Autodesk Inventor part; units mm, degrees
ref_plane "YZ Plane" through (0, 0, 0) normal (1, 0, 0) x (0, 1, 0)
ref_plane "XZ Plane" through (0, 0, 0) normal (0, 1, 0) x (-1, 0, 0)
ref_plane "XY Plane" through (0, 0, 0) normal (0, 0, 1) x (1, 0, 0)
ref_plane "作業平面1" through (15.3757, 45.25, -5) normal (0, 0, -1) x (-1, 0, 0)
sketch "Base_plate" plane through (15.3757, 45.25, -5) normal (0, 0, -1) x (-1, 0, 0)
  circle A0 centre (-112.6243, -12.25) radius 3.25
  circle A1 centre (-112.6243, -78.25) radius 3.25
  circle A2 centre (143.3757, -78.25) radius 3.25
  circle A3 centre (143.3757, -12.25) radius 3.25
  line L0 (151.578, -11.3644) -> (151.578, -77.3644)
  arc A4 (151.578, -11.3644) -> (147.5007, -5.1053) centre (143.3757, -12.25) ccw
  line L1 (147.5007, -5.1053) -> (140.9785, -1.3397)
  arc A5 (140.9785, -1.3397) -> (135.9785, 0) centre (135.9785, -10) ccw
  line L2 (135.9785, 0) -> (0, 0)
  line L3 (-20.2421, 7.2915) -> (-3.697, 0.7085)
  line L4 (-23.9391, 8) -> (-103.3743, 8)
  line L5 (0, 0) -> (135.9785, 0)
  arc A6 (140.9785, -1.3397) -> (135.9785, 0) centre (135.9785, -10) ccw
  line L6 (140.9785, -1.3397) -> (147.5007, -5.1053)
  arc A7 (151.578, -11.3644) -> (147.5007, -5.1053) centre (143.3757, -12.25) ccw
  line L7 (151.578, -11.3644) -> (151.578, -77.3644)
  arc A8 (147.5007, -85.3947) -> (151.578, -77.3644) centre (143.3757, -78.25) ccw
  arc A9 (-103.3743, 8) -> (-111.5876, 3.7046) centre (-103.3743, -2) ccw
  line L8 (-103.3743, 8) -> (-23.9391, 8)
  arc A10 (-20.2421, 7.2915) -> (-23.9391, 8) centre (-23.9391, -2) ccw
  line L9 (-20.2421, 7.2915) -> (-3.697, 0.7085)
  arc A11 (-3.697, 0.7085) -> (0, 0) centre (0, 10) ccw
  circle A12 centre (-112.6243, -12.25) radius 3.25
  circle A13 centre (143.3757, -12.25) radius 3.25
  circle A14 centre (143.3757, -78.25) radius 3.25
  circle A15 centre (-112.6243, -78.25) radius 3.25
  line L10 (135.9785, 0) -> (0, 0)
  arc A16 (140.9785, -1.3397) -> (135.9785, 0) centre (135.9785, -10) ccw
  line L11 (147.5007, -5.1053) -> (140.9785, -1.3397)
  arc A17 (151.578, -11.3644) -> (147.5007, -5.1053) centre (143.3757, -12.25) ccw
  line L12 (151.6257, -11.3644) -> (151.6257, -77.3644)
  arc A18 (147.5007, -85.3947) -> (151.578, -77.3644) centre (143.3757, -78.25) ccw
  line L13 (147.5007, -85.3947) -> (140.9785, -89.1603)
  arc A19 (135.9785, -90.5) -> (140.9785, -89.1603) centre (135.9785, -80.5) ccw
  line L14 (135.9785, -90.5) -> (0, -90.5)
  arc A20 (0, -90.5) -> (-3.697, -91.2085) centre (0, -100.5) ccw
  line L15 (-20.2421, -97.7915) -> (-3.697, -91.2085)
  arc A21 (-23.9391, -98.5) -> (-20.2421, -97.7915) centre (-23.9391, -88.5) ccw
  line L16 (-23.9391, -98.5) -> (-103.3743, -98.5)
  arc A22 (-111.5876, -94.2046) -> (-103.3743, -98.5) centre (-103.3743, -88.5) ccw
  line L17 (-111.5876, -94.2046) -> (-119.4003, -82.9563)
  arc A23 (-120.8743, -78.25) -> (-119.4003, -82.9563) centre (-112.6243, -78.25) ccw
  line L18 (-120.8743, -12.25) -> (-120.8743, -78.25)
  arc A24 (-119.4003, -7.5437) -> (-120.8743, -12.25) centre (-112.6243, -12.25) ccw
  line L19 (-111.5876, 3.7046) -> (-119.4003, -7.5437)
  line L20 (-23.9391, 8) -> (-103.3743, 8)
  arc A25 (-20.2421, 7.2915) -> (-23.9391, 8) centre (-23.9391, -2) ccw
  line L21 (-20.2421, 7.2915) -> (-3.697, 0.7085)
  arc A26 (-3.697, 0.7085) -> (0, 0) centre (0, 10) ccw
  line L22 (101.578, 7.8213) -> (101.578, -100.5) construction
  line L23 (151.6257, -44.3644) -> (-114.4175, -44.3644) construction
  circle A27 centre (56.078, -44.3644) radius 17.5 construction
  line L24 (129.578, -5.1053) -> (129.578, -82.9563) construction
  circle A28 centre (129.578, -16.3644) radius 1.75
  circle A29 centre (129.578, -72.3644) radius 1.75
  line L25 (59.578, -19.3302) -> (59.578, -75) construction
  circle A30 centre (59.578, -24.3644) radius 1.75
  circle A31 centre (59.578, -64.3644) radius 1.75
  circle A32 centre (101.578, -44.3644) radius 14.75 construction
  line L26 (101.578, -44.3644) -> (118.6401, -27.3023) construction
  line L27 (101.578, -44.3644) -> (125.7075, -44.3644) construction
  line L28 (106.5779, -39.3645) -> (117.1845, -28.7579) construction
  line L29 (107.7093, -40.4959) -> (118.3159, -29.8893)
  line L30 (116.0532, -27.6265) -> (105.4466, -38.2331)
  arc A33 (105.4466, -38.2331) -> (107.7093, -40.4959) centre (106.5779, -39.3645) ccw
  arc A34 (118.3159, -29.8893) -> (116.0532, -27.6265) centre (117.1845, -28.7579) ccw
  line L31 (84.8401, -29.8893) -> (95.4467, -40.4959)
  arc A35 (87.1028, -27.6265) -> (84.8401, -29.8893) centre (85.9714, -28.7579) ccw
  line L32 (97.7094, -38.2331) -> (87.1028, -27.6265)
  arc A36 (95.4467, -40.4959) -> (97.7094, -38.2331) centre (96.578, -39.3645) ccw
  line L33 (87.1028, -61.1024) -> (97.7094, -50.4958)
  arc A37 (84.8401, -58.8396) -> (87.1028, -61.1024) centre (85.9714, -59.971) ccw
  line L34 (95.4467, -48.233) -> (84.8401, -58.8396)
  arc A38 (97.7094, -50.4958) -> (95.4467, -48.233) centre (96.578, -49.3644) ccw
  line L35 (118.3159, -58.8396) -> (107.7093, -48.233)
  arc A39 (116.0532, -61.1024) -> (118.3159, -58.8396) centre (117.1845, -59.971) ccw
  line L36 (105.4466, -50.4958) -> (116.0532, -61.1024)
  arc A40 (107.7093, -48.233) -> (105.4466, -50.4958) centre (106.5779, -49.3644) ccw
  line L37 (65.0919, -29.3644) -> (74.078, -29.3644)
  line L38 (84.078, -39.3644) -> (84.078, -49.3644)
  line L39 (74.078, -59.3644) -> (65.0919, -59.3644)
  line L40 (65.0919, -59.3644) -> (65.0919, -29.3644) construction
  arc A41 (84.078, -39.3644) -> (74.078, -29.3644) centre (74.078, -39.3644) ccw
  arc A42 (74.078, -59.3644) -> (84.078, -49.3644) centre (74.078, -49.3644) ccw
  arc A43 (65.0919, -29.3644) -> (65.0919, -59.3644) centre (56.078, -44.3644) ccw
  line L41 (-60.8743, -12.5765) -> (-60.8743, -79.1684) construction
  line L42 (-98.3743, -6.8644) -> (-23.3743, -6.8644) construction
  line L43 (-23.3743, -6.8644) -> (-23.3743, -81.8644) construction
  line L44 (-23.3743, -81.8644) -> (-98.3743, -81.8644) construction
  line L45 (-98.3743, -81.8644) -> (-98.3743, -6.8644) construction
  line L46 (-98.3743, -6.8644) -> (-23.3743, -81.8644) construction
  line L47 (-23.3743, -6.8644) -> (-98.3743, -81.8644) construction
  circle A44 centre (-98.3743, -6.8644) radius 2.1
  circle A45 centre (-23.3743, -6.8644) radius 2.1
  circle A46 centre (-98.3743, -81.8644) radius 2.1
  circle A47 centre (-23.3743, -81.8644) radius 2.1
  point P0 (144.2396, -3.2225)
  point P1 (144.2396, -87.2775)
  point P2 (111.8812, -34.0612)
  point P3 (91.2747, -34.0612)
  point P4 (91.2747, -54.6677)
  point P5 (111.8812, -54.6677)
  point P6 (-60.8743, -44.3644)
  point P7 (-60.8743, -44.3644)
  dimension "d20" = 50
  dimension "d21" = 45.5
  dimension "d22" = 35
  dimension "d23" = 28
  dimension "d24" = 3.5
  dimension "d25" = 3.5
  dimension "d26" = 28
  dimension "d27" = 28
  dimension "d28" = 42
  dimension "d29" = 3.5
  dimension "d30" = 3.5
  dimension "d31" = 20
  dimension "d32" = 20
  dimension "d40" = 29.5
  dimension "d43" = 45
  dimension "d44" = 3.2
  dimension "d45" = 7.071
  dimension "d46" = 15
  dimension "d49" = 360
  dimension "d51" = 15
  dimension "d52" = 15
  dimension "d53" = 28
  dimension "d54" = 10
  dimension "d65" = 60
  dimension "d66" = 75
  dimension "d67" = 75
  dimension "d68" = 4.2
  dimension "d69" = 4.2
  dimension "d70" = 4.2
  dimension "d71" = 4.2
sketch "RPLidarA1M8" plane through (15.3757, 45.25, -5) normal (0, 0, -1) x (-1, 0, 0)
  line L0 (59.578, -45.9195) -> (59.578, -117.33) construction
  circle A0 centre (59.578, -24.3644) radius 1.5
  circle A1 centre (59.578, -64.3644) radius 1.5
  line L1 (4.0197, -44.3644) -> (199.1363, -44.3644) construction
  circle A2 centre (129.578, -16.3644) radius 1.5
  line L2 (101.578, -2.732) -> (101.578, -85.9969) construction
  circle A3 centre (101.578, -44.3644) radius 35.14
  line L3 (59.578, -6.852) -> (59.578, -81.8768) construction
  circle A4 centre (129.578, -72.3644) radius 1.5
  line L4 (129.578, -10.2254) -> (129.578, -77.75) construction
  circle A5 centre (56.078, -44.3644) radius 10
  circle A6 centre (56.078, -44.3644) radius 16
  line L5 (151.6257, -44.3644) -> (-114.4175, -44.3644) construction
  line L6 (101.578, 7.8213) -> (101.578, -100.5) construction
  point P0 (15.3757, -88.1377)
  point P1 (59.578, -44.3644)
  point P2 (129.578, -43.9877)
  dimension "d1" = 3
  dimension "d2" = 3
  dimension "d5" = 20
  dimension "d6" = 3
  dimension "d10" = 70.28
  dimension "d11" = 42
  dimension "d12" = 40
  dimension "d13" = 3
  dimension "d14" = 28
  dimension "d15" = 28
  dimension "d16" = 28
  dimension "d17" = 20
  dimension "d18" = 45.5
  dimension "d19" = 32
sketch "RPLidarA2M6" plane through (15.3757, 45.25, -5) normal (0, 0, -1) x (-1, 0, 0)
  line L0 (101.578, 7.8213) -> (101.578, -100.5) construction
  line L1 (151.6257, -44.3644) -> (-114.4175, -44.3644) construction
  circle A0 centre (101.578, -44.3644) radius 14.75 construction
  circle A1 centre (112.0078, -33.9346) radius 1.5
  line L2 (112.0078, -33.9346) -> (101.578, -44.3644) construction
  circle A2 centre (91.1482, -33.9346) radius 1.5
  circle A3 centre (91.1482, -54.7943) radius 1.5
  circle A4 centre (112.0078, -54.7943) radius 1.5
  dimension "d33" = 29.5
  dimension "d34" = 3
  dimension "d35" = 45
  dimension "d38" = 360
extrude "押し出し1" add sketch "Base_plate" along normal blind 5
Read the model definition and answer for the solid it produces. Units are mm, in the model's axes. A direction names the side the tool comes from. Coordinates: 2 decimals unless noted, no trailing zeros. Loops run counter-clockwise (first coordinate to the right, second up) from the corner with the lowest first, then second, coordinate; pieces in that order, holes last. Notation, with made-up numbers: (-17.5, -37) -> (-1.5, -37) arc R17 cw to (-1.5, -21) -> close; hole circle Ø9 at (81.25, 51). An arc over 180 degrees is marked (long way). Write item = value, one per line. Start each with the question number.
1) The part is cut by section B-B, the plane y = 11.5. Determine the outline of the cut face in (x, z), plus the area to 3 significant figures.
2) The mould has two halves that part along Y. Classify faces 1 (the face through (-134.88, 37.55, -7.46)), 2 (the face through (-131.002, -31.755, -7.465)), 3 (the face through (27.461, -49.296, -7.465)): pulls with the +Y half, pulls with the -Y half, needs draft (parallel to the pull), parting line crosses it, or undercut.
3) The part is cut by section A-A, the plane x = -128. Determine the outline of the cut face in (y, z).
4) Given P1, Ø4, axis at x = -128, y = 33, coming from the -Z side; P2, Ø5, axis at x = 38.75, y = 38.39, coming from the +Z side; P3, Ø2.5, axis at x = -28, z = -8.5, coming from the -Y side; P4, Ø2, axis at x = 12.5, z = -9, coming from the +Y side, each flat-ended and moving along its own axis, determine where each tip first touches the part or whether it passes through.
5) The part is cut by section C-C, the plane x = -28.5. Determine the outline of the cut face in (y, z), plus the area to 3 significant figures.
6) For faces 4 (the face through (-68.702, 1, -7)), 5 (the face through (-123.156, 44.919, -7.465)), determine the directions among +Z, -Z, +X, -X, +Y, -Y from which every point of the face is accessible in a straight line to the end or side of a thin tool.
7) Find the intervals of material crossed by L1, parallel to Y at x = 113.75, z = -6.4; L2, parallel to Y at x = -101, z = -7.1; L3, parallel to X at y = -6, z = -9.25, in increasing order. Write a range as from..to.
8) The part is cut by section D-D, the plane z = -6.75. State how many separate pieces and enclosed holes the cut face has, plus the area to 3 significant figures.
Result:
q1.outline = (-136.2, -10) -> (-99.08, -10) -> (-99.08, -5) -> (-136.2, -5) -> close; (-94.55, -10) -> (-77.85, -10) -> (-77.85, -5) -> (-94.55, -5) -> close; (-73.33, -10) -> (-66.98, -10) -> (-66.98, -5) -> (-73.33, -5) -> close; (-26.79, -10) -> (136.25, -10) -> (136.25, -5) -> (-26.79, -5) -> close
q1.area = 1,120 mm²
q2.face_1 = pulls with the +Y half
q2.face_2 = undercut
q2.face_3 = pulls with the -Y half
q3.outline = (-42.53, -10) -> (-36.25, -10) -> (-36.25, -5) -> (-42.53, -5) -> close; (-29.75, -10) -> (29.75, -10) -> (29.75, -5) -> (-29.75, -5) -> close; (36.25, -10) -> (42.53, -10) -> (42.53, -5) -> (36.25, -5) -> close
q4.P1 = through
q4.P2 = -5
q4.P3 = -45.25
q4.P4 = 45.25
q5.outline = (-45.25, -10) -> (-11.66, -10) -> (-11.66, -5) -> (-45.25, -5) -> close; (13.43, -10) -> (45.25, -10) -> (45.25, -5) -> (13.43, -5) -> close
q5.area = 327 mm²
q6.face_4 = +Z, -Z
q6.face_5 = +Z, -Z, -X, +Y
q7.L1 = -53.25..-38.71, -34.51..36.29, 40.49..53.25
q7.L2 = -45.25..-16.1, -11.65..13.42, 17.87..45.25
q7.L3 = -136.2..-95.35, -90.83..-81.58, -77.05..-68.52, -24.61..136.25
q8.separate_pieces = 1
q8.enclosed_holes = 17
q8.area = 24,300 mm²
